```python
from build123d import *

# Parameters (mm, degrees)
F0_W     = 57.15
F0_H     = 38.1
F1_DEPTH = 12.7
F3_DEPTH = 12.7
F4_R     = 10.090212
F5_DEPTH = 25.4


with BuildPart() as f1:
    # F0 (on Front) → F1 (new body)
    with BuildSketch(Plane.XZ):
        with Locations((28.575, 19.05)):
            Rectangle(F0_W, F0_H)
    extrude(amount=F1_DEPTH)

    # F2 (on face) → F3 (join)
    with BuildSketch(Plane.XZ.offset(12.7)):
        Polygon((19.05, 38.1), (0, 38.1), (0, 0), (44.45, 0), align=None)
    extrude(amount=F3_DEPTH)

    # F4 (on face) → F5 (cut)
    with BuildSketch(Plane.XZ.offset(25.4)):
        with Locations((31.75, 19.05)):
            Circle(F4_R)
    extrude(amount=-F5_DEPTH, mode=Mode.SUBTRACT)


solid = f1.part
```
Design review of the part built by this model. Coordinates are the model's own, in mm. A direction names the side the tool comes from. Coordinates: 2 decimals unless noted, no trailing zeros. Order: outer loops, then holes, each group sorted by start corner. A loop starts at its lowest first (then second) coordinate and runs counter-clockwise, first axis right, second up. Notation, with made-up numbers: M 83.5,-24 L 132.5,-24 A12 ccw 132.5,-8 Z; hole C 67.5,-39 d7. An arc over 180 degrees is marked long. Answer as a JSON object with one key per item and string values. Group by question number.
1) Mouldability with a two-part tool opening along Z and no side actions: class faces 3 (the flat face through (28, -13, 0)), 4 (the cylindrical face through (23.743, -10.056, 12.91)), 5 (the flat face through (22.65, -18.96, 32.7)) as pulls with the +Z half, pulls with the -Z half, needs draft (parallel to the pull), parting line crosses it, or undercut.
2) Add section C-C, the plane y = -7.5. Write out the cut boundary in (x, z).
3) Add section D-D, the plane y = -14.75. Write out the cut boundary in (x, z).
4) Add section A-A, the plane x = 31.75. Write out the cut boundary in (y, z), then the cut area to 3 significant figures.
5) For pin 1 (1.5 mm diameter, centred on y = -19.5, z = 7.5, fed in from +X); pin 2 (8 mm diameter, centred on x = 45, z = 14, fed in from +Y); pin 3 (6 mm diameter, centred on x = 47.5, z = 13.5, fed in from -Y), all flat-tipped, find the tip position at first contact; note any pin that passes through.
6) Wall thickness on L1, parallel to X at y = -9.25, z = 19.05; L2, parallel to Z at x = 31.75, y = -11.5; L3, parallel to Y at x = 48, z = 14: over which ranges is each line inside the solid? List them lowest first.
7) Tool access review of faces 1 (the flat face through (46, -12.7, 24)), 2 (the flat face through (22, 0, 24)): name each direction out of +Z, -Z, +X, -X, +Y, -Y from which nothing blocks a thin tool from reaching the whole face with its end or side.
8) Add section B-B, the plane z = 19.05. Write out the cut boundary in (x, y).
Computed values:
{
 "1": {"face 3": "pulls with the -Z half", "face 4": "undercut", "face 5": "pulls with the +Z half"},
 "2": {"outline": "M 0,0 L 57.15,0 L 57.15,38.1 L 0,38.1 Z; hole C 31.75,19.05 d20.18"},
 "3": {"outline": "M 0,0 L 44.45,0 L 37.35,10.65 A10.09 cw 26.15,27.45 L 19.05,38.1 L 0,38.1 Z"},
 "4": {"outline": "M -25.4,0 L 0,0 L 0,8.96 L -25.4,8.96 Z; M -12.7,29.14 L 0,29.14 L 0,38.1 L -12.7,38.1 Z", "area": "341 mm^2"},
 "5": {"pin 1": "stops at x = 39.95", "pin 2": "stops at y = 0", "pin 3": "stops at y = -12.7"},
 "6": {"L1": "x = 0 to 21.66, 41.84 to 57.15", "L2": "z = 0 to 8.96, 29.14 to 38.1", "L3": "y = -12.7 to 0"},
 "7": {"face 1": "+Z, +X, -Y", "face 2": "+Z, -Z, +X, -X, +Y"},
 "8": {"outline": "M 0,-25.4 L 21.66,-25.4 L 21.66,0 L 0,0 Z; M 41.84,-12.7 L 57.15,-12.7 L 57.15,0 L 41.84,0 Z"}
}
